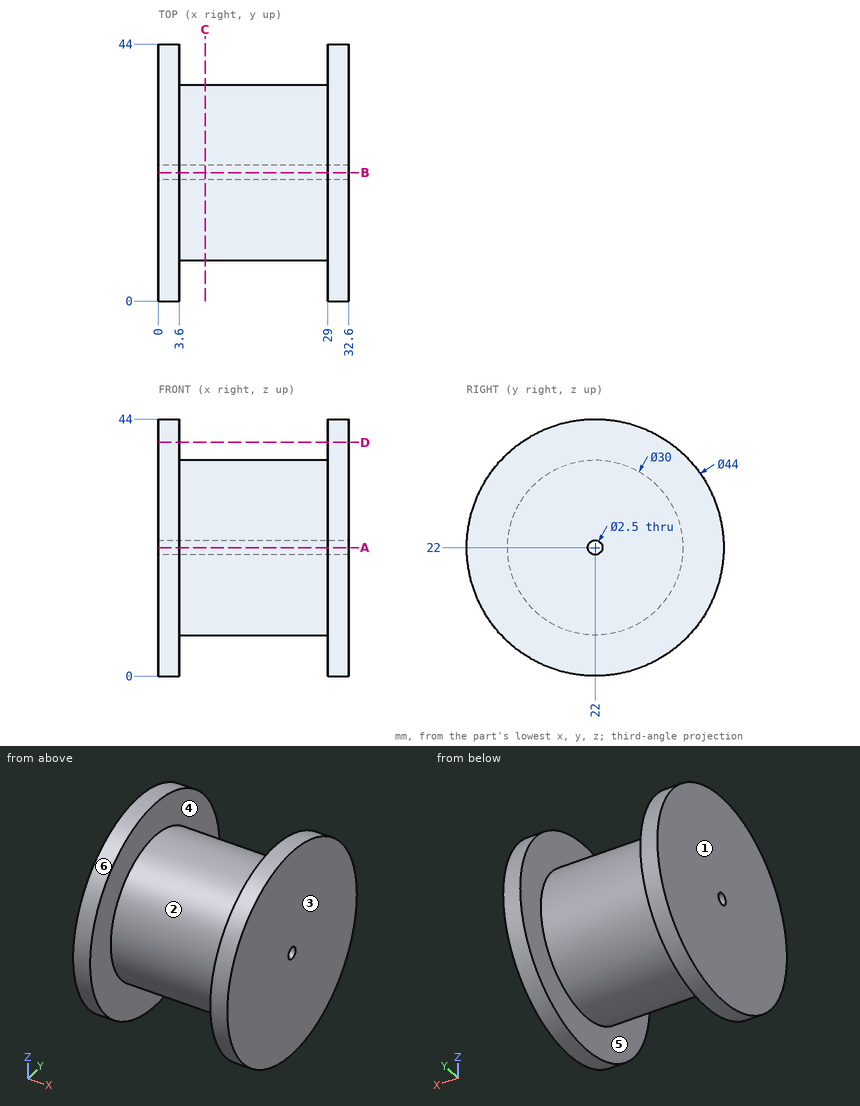
Could you check a few things on this drawing? It's one solid part, dimensions in mm from its lowest x, y, z. A direction names the side the tool comes from. Give positions to 0.01 mm unless a question says otherwise; leave off trailing zeros. Order: outer loops, then holes, each group sorted by start corner. A loop starts at its lowest first (then second) coordinate and runs counter-clockwise, first axis right, second up. Notation, with made-up numbers: (84.25, 29) - (102.25, 29) arc R20 cw to (102.25, 56) - close; hole circle Ø3 at (-6.5, 77.5). An arc over 180 degrees is marked (long way). Answer as a JSON object with one key per item and string values. Group by question number.
Item 1: If we mould it in two halves opening along X, with no side actions, what happens to the marked faces 3, 4, 5 and 6? For each: pulls with the +X half, pulls with the -X half, needs draft (parallel to the pull), parting line crosses it, or undercut.
Item 2: Please list where these lines run through material, in increasing order: probe 1 along X at (y, z) = (16, 5.5); probe 2 along Y at (x, z) = (16, 22); probe 3 along Z at (x, y) = (24, 22.5).
Item 3: If we section it at D-D on z = 40: Please give me the cut outline in (x, y).
Item 4: For P1, Ø1.5, axis at x = 27.5, z = 39, coming from the -Y side; P2, Ø1.5, axis at x = 15.5, y = 22, coming from the -Z side; P3, Ø4, axis at x = 14, y = 15.5, coming from the +Z side, each with a flat end and sliding along its axis, tell me the tip position at first contact or that it passes through.
Item 5: If we section it at C-C on x = 8: Please give me the cut outline in (y, z), and give its area (3 significant figures).
Item 6: If we section it at A-A on z = 22: Please give me the cut outline in (x, y).
Item 7: Which directions (+Z, -Z, +X, -X, +Y, -Y) give clear straight access to the entire face, cutting with the end or side of a thin tool? Please do the marked faces 1 and 2.
Result set:
{
 "1": {"face 3": "pulls with the +X half", "face 4": "undercut", "face 5": "undercut", "face 6": "needs draft"},
 "2": {"probe 1": "0 to 3.6, 29 to 32.6", "probe 2": "7 to 20.75, 23.25 to 37", "probe 3": "7.01 to 20.85, 23.15 to 36.99"},
 "3": {"outline": "(0, 9.35) - (3.6, 9.35) - (3.6, 34.65) - (0, 34.65) - close; (29, 9.35) - (32.6, 9.35) - (32.6, 34.65) - (29, 34.65) - close"},
 "4": {"P1": "through", "P2": "z = 7", "P3": "z = 36.31"},
 "5": {"outline": "circle Ø30 at (22, 22); hole circle Ø2.5 at (22, 22)", "area": "702 mm²"},
 "6": {"outline": "(0, 0) - (3.6, 0) - (3.6, 7) - (29, 7) - (29, 0) - (32.6, 0) - (32.6, 20.75) - (0, 20.75) - close; (0, 23.25) - (32.6, 23.25) - (32.6, 44) - (29, 44) - (29, 37) - (3.6, 37) - (3.6, 44) - (0, 44) - close"},
 "7": {"face 1": "+Z, -Z, -X, +Y, -Y", "face 2": "none"}
}
